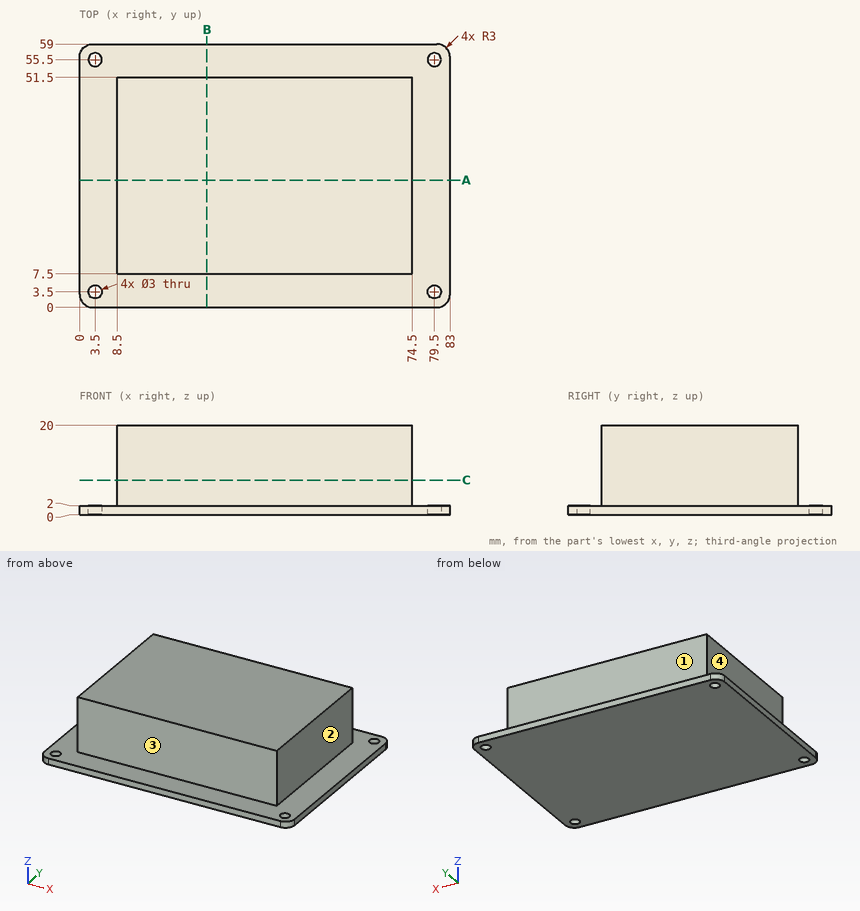
Source: three-view drawing plus pictorial views. Frame: mm from the lowest corner of the part. A direction names the side the tool comes from. Round coordinates to 2 decimals unless told otherwise and drop trailing zeros. Loops run counter-clockwise (first coordinate to the right, second up) from the corner with the lowest first, then second, coordinate; pieces in that order, holes last.
Q1. Section C-C, the plane z = 7.75. Return loops of the section in (x, y).
Q2. Section B-B, the plane x = 28.5. Return loops of the section in (y, z), plus the area to 3 significant figures.
Q3. Section A-A, the plane y = 28.5. Return loops of the section in (x, z), plus the area to 3 significant figures.
Q4. Ray query, line 1 (Y direction, x = 3.5, z = 1.65); line 2 (Z direction, x = 53.5, y = 5.5); line 3 (Y direction, x = 32.5, z = 7). Return the intervals inside material, ascending.
Q5. Access query for the marked faces 1, 2, 3 and 4. Directions: +Z, -Z, +X, -X, +Y, -Y. A direction counts if a zero-diameter tool reaches every point of the face in a straight line with its end or side. Return the directions, or none.
Q6. First-contact query: P1, Ø5, axis at x = 33.5, y = 37.5, coming from the -Z side; P2, Ø9, axis at y = 19, z = 7.5, coming from the -X side; P3, Ø5, axis at x = 79.5, y = 55.5, coming from the +Z side; P4, Ø10, axis at x = 61, z = 8, coming from the -Y side. Flat tips, straight axial feed; report the tip coordinate or a pass-through.
Solutions:
1. outline: (8.5, 7.5) - (74.5, 7.5) - (74.5, 51.5) - (8.5, 51.5) - close
2. outline: (0, 0) - (59, 0) - (59, 2) - (51.5, 2) - (51.5, 20) - (7.5, 20) - (7.5, 2) - (0, 2) - close
2. area: 910 mm2
3. outline: (0, 0) - (83, 0) - (83, 2) - (74.5, 2) - (74.5, 20) - (8.5, 20) - (8.5, 2) - (0, 2) - close
3. area: 1,350 mm2
4. line 1: y = 0 to 2, 5 to 54, 57 to 59
4. line 2: z = 0 to 2
4. line 3: y = 7.5 to 51.5
5. face 1: +Z, +X, -X, +Y
5. face 2: +Z, +X, +Y, -Y
5. face 3: +Z, +X, -X, -Y
5. face 4: +Z, -X, +Y, -Y
6. P1: stops at z = 0
6. P2: stops at x = 8.5
6. P3: stops at z = 2
6. P4: stops at y = 7.5
